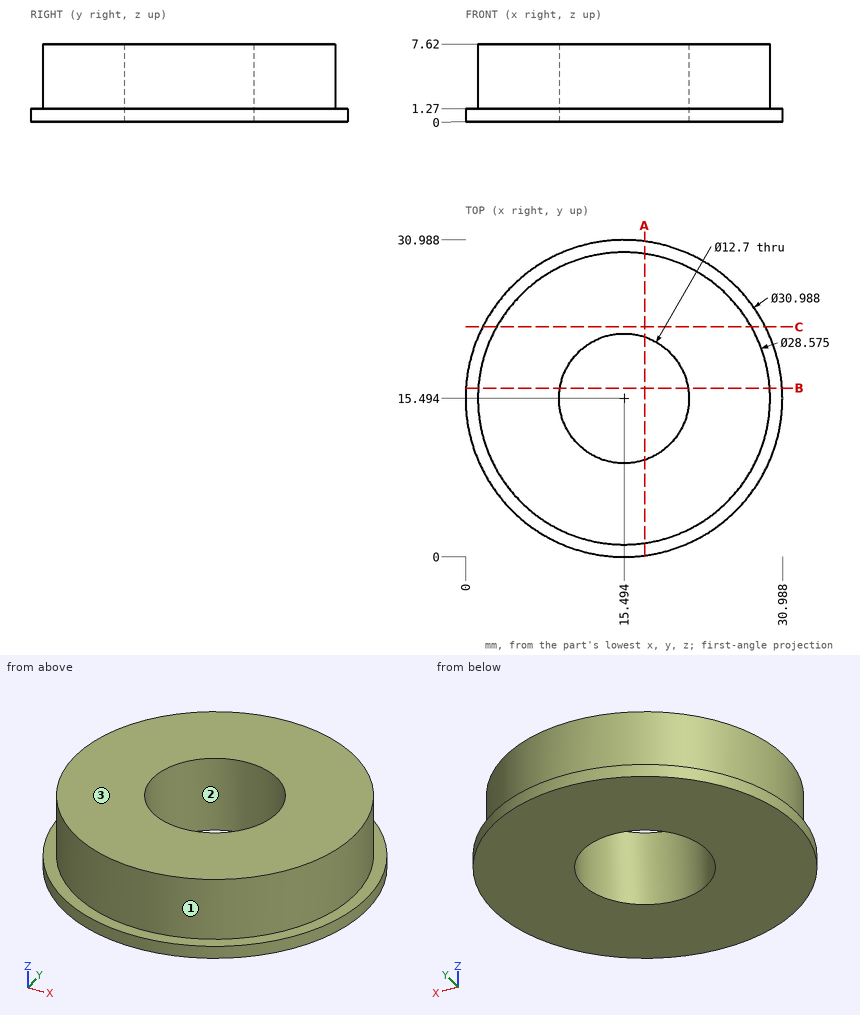
Geometry check sheet. Reference: drawing and pictorial views, mm from the part's lowest x, y, z. Give positions to 0.01 mm unless a question says otherwise; leave off trailing zeros. Loops run counter-clockwise (first coordinate to the right, second up) from the corner with the lowest first, then second, coordinate; pieces in that order, holes last.
1. Go/stop test with a flat-tipped pin: pin 1 Ø4 at (y, z) = (27.5, 6) entering from -X. Record where the tip stops, or that it passes through.
2. Section check B-B, the plane y = 16.5. Enter the section's corners in (x, z).
3. Section check C-C, the plane y = 22.5. Enter the section's corners in (x, z), then the cut area to 3 significant figures.
4. Mould release check, pull along Y, two halves, no side actions. Record for the marked faces 1, 2 and 3: released by +Y, released by -Y, zero draft, split by the parting line, or undercut.
5. Section check A-A, the plane x = 17.5. Enter the section's corners in (y, z), then the cut area to 3 significant figures.
6. Thickness scan on line 1 (Z direction, x = 12.5, y = 29.5); line 2 (Y direction, x = 14.5, z = 4.25); line 3 (X direction, y = 19, z = 3). Record the ranges inside material, lowest first.
Geometry says:
1. pin 1: stops at x = 5.3
2. outline: (0.03, 0) - (9.22, 0) - (9.22, 7.62) - (1.24, 7.62) - (1.24, 1.27) - (0.03, 1.27) - close; (21.76, 0) - (30.96, 0) - (30.96, 1.27) - (29.75, 1.27) - (29.75, 7.62) - (21.76, 7.62) - close
3. outline: (1.67, 0) - (29.31, 0) - (29.31, 1.27) - (27.95, 1.27) - (27.95, 7.62) - (3.04, 7.62) - (3.04, 1.27) - (1.67, 1.27) - close
3. area: 193 mm2
4. face 1: split by the parting line
4. face 2: undercut
4. face 3: zero draft
5. outline: (0.13, 0) - (9.47, 0) - (9.47, 7.62) - (1.35, 7.62) - (1.35, 1.27) - (0.13, 1.27) - close; (21.52, 0) - (30.86, 0) - (30.86, 1.27) - (29.64, 1.27) - (29.64, 7.62) - (21.52, 7.62) - close
5. area: 127 mm2
6. line 1: z = 0 to 1.27
6. line 2: y = 1.24 to 9.22, 21.77 to 29.75
6. line 3: x = 1.64 to 10.2, 20.79 to 29.34
